from build123d import *

# Parameters (mm, degrees)
SKETCH1_W           = 230
SKETCH1_H           = 102
BOSS_EXTRUDE1_DEPTH = 2
SKETCH2_W           = 37
SKETCH2_H           = 22
SKETCH2_W_2         = 35
SKETCH2_H_2         = 9
SKETCH2_W_3         = 50
SKETCH2_H_3         = 56
CUT_EXTRUDE1_DEPTH  = 252.610810579
SKETCH3_R           = 1.65
CUT_EXTRUDE2_DEPTH  = 10
FILLET1_R           = 4
FILLET2_SIZE        = 4
FILLET2_SIZE_2      = 12
FILLET3_R           = 10
SKETCH4_R           = 1.65
CUT_EXTRUDE3_DEPTH  = 10


with BuildPart() as part:
    # Sketch1 → Boss-Extrude1 (new body)
    with BuildSketch(Plane(origin=(0, 0, 0), x_dir=(1, 0, 0), z_dir=(0, 1, 0))):
        with Locations((115, 51)):
            Rectangle(SKETCH1_W, SKETCH1_H)
    extrude(amount=BOSS_EXTRUDE1_DEPTH)

    # Sketch2 → Cut-Extrude1 (cut, through all)
    with BuildSketch(Plane(origin=(0, 2, 0), x_dir=(1, 0, 0), z_dir=(0, 1, 0))):
        with Locations((18.5, 91)):
            Rectangle(SKETCH2_W, SKETCH2_H)
        with Locations((17.5, 4.5)):
            Rectangle(SKETCH2_W_2, SKETCH2_H_2)
        with Locations((211.5, 91)):
            Rectangle(SKETCH2_W, SKETCH2_H)
        with Locations((212.5, 4.5)):
            Rectangle(SKETCH2_W_2, SKETCH2_H_2)
        with Locations((115, 28)):
            Rectangle(SKETCH2_W_3, SKETCH2_H_3)
    extrude(amount=-CUT_EXTRUDE1_DEPTH, mode=Mode.SUBTRACT)

    # Sketch3 → Cut-Extrude2 (cut)
    with BuildSketch(Plane.XZ):
        with Locations(Location((5, -14, 0), (0, 0, 270))):
            Circle(SKETCH3_R)
        with Locations(Location((5, -75, 0), (0, 0, 270))):
            Circle(SKETCH3_R)
        with Locations(Location((95, -59.5, 0), (0, 0, 270))):
            Circle(SKETCH3_R)
        with Locations(Location((135, -59.5, 0), (0, 0, 270))):
            Circle(SKETCH3_R)
        with Locations(Location((225, -14, 0), (0, 0, 270))):
            Circle(SKETCH3_R)
        with Locations(Location((225, -75, 0), (0, 0, 270))):
            Circle(SKETCH3_R)
    extrude(amount=-CUT_EXTRUDE2_DEPTH, mode=Mode.SUBTRACT)

    # Fillet1
    fillet1_edges = [part.edges().sort_by_distance(p)[0] for p in [
        (0, 1, -9),
        (230, 1, -80),
        (230, 1, -9),
        (90, 1, 0),
        (140, 1, 0),
        (0, 1, -80),
    ]]
    fillet(fillet1_edges, radius=FILLET1_R)

    # Fillet2
    # an asymmetric fillet: 12, 4 mm, written as the material it adds along each edge
    with BuildSketch(Plane(origin=(195, 2, -9), x_dir=(0, 0, 1), z_dir=(0, -1, 0))) as fillet2_piece_1:
        with BuildLine():
            Bezier((FILLET2_SIZE, 0), (0, 0), (0, -FILLET2_SIZE_2), weights=[1, 0.707106781, 1])
            Line((0, -FILLET2_SIZE_2), (0, 0))
            Line((0, 0), (FILLET2_SIZE, 0))
        make_face()
    extrude(amount=2)
    with BuildSketch(Plane(origin=(35, 2, -9), x_dir=(0, 0, 1), z_dir=(0, -1, 0))) as fillet2_piece_2:
        with BuildLine():
            Bezier((FILLET2_SIZE, 0), (0, 0), (0, FILLET2_SIZE_2), weights=[1, 0.707106781, 1])
            Line((0, FILLET2_SIZE_2), (0, 0))
            Line((0, 0), (FILLET2_SIZE, 0))
        make_face()
    extrude(amount=2)

    # Fillet3
    fillet3_edges = [part.edges().sort_by_distance(p)[0] for p in [
        (35, 1, 0),
        (195, 1, 0),
    ]]
    fillet(fillet3_edges, radius=FILLET3_R)

    # Sketch4 → Cut-Extrude3 (cut)
    with BuildSketch(Plane.XZ):
        with Locations(Location((61, -7, 0), (0, 0, 270))):
            Circle(SKETCH4_R)
        with Locations(Location((169, -7, 0), (0, 0, 270))):
            Circle(SKETCH4_R)
    extrude(amount=-CUT_EXTRUDE3_DEPTH, mode=Mode.SUBTRACT)


solid = part.part
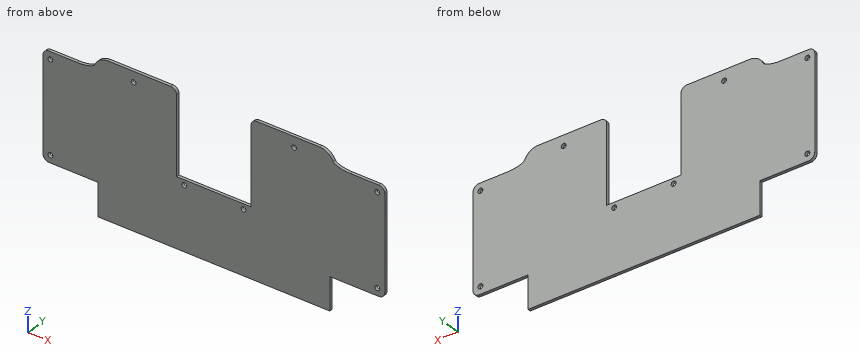
Read the model definition and answer for the solid it produces. Units are mm, in the model's axes. Round coordinates to 2 decimals unless told otherwise and drop trailing zeros. Write each loop counter-clockwise with the first axis right and the second up, starting at its lowest first coordinate (ties: lowest second). Pieces come first, ordered by that corner, then holes.
1. The part is cut by section B-B, the plane y = 1. State how many separate pieces and enclosed holes the cut face has, then the cut area to 3 significant figures.
2. The part is cut by section A-A, the plane z = -19.5. Determine the outline of the cut face in (x, y).
3. The part is cut by section C-C, the plane x = 114. Determine the outline of the cut face in (y, z), then the cut area to 3 significant figures.
4. Given pin 1 Ø0.6 at (x, y) = (219.5, 1.5) entering from +Z; pin 2 Ø1 at (x, y) = (27.5, 0.5) entering from -Z; pin 3 Ø0.6 at (y, z) = (0.5, -88) entering from -X, each flat-ended and moving along its own axis, determine where each tip first touches the part or whether it passes through.
5. Straight lines are drawn through the part: L1, parallel to X at y = 1.5, z = -75; L2, parallel to X at y = 1, z = -14; L3, parallel to Z at x = 225, y = 1.05. For each, find the intervals that lie inside material, in ascending order.
6. The part is cut by section D-D, the plane z = -88. Determine the outline of the cut face in (x, y), then the cut area to 3 significant figures.
Values:
1. separate pieces: 1
1. enclosed holes: 8
1. area: 18,300 mm2
2. outline: (0, 0) - (90, 0) - (90, 2) - (0, 2) - close; (140, 0) - (230, 0) - (230, 2) - (140, 2) - close
3. outline: (0, -102) - (2, -102) - (2, -56) - (0, -56) - close
3. area: 92.0 mm2
4. pin 1: stops at z = -9
4. pin 2: stops at z = -80
4. pin 3: stops at x = 37
5. L1: x = 0 to 3.35, 6.65 to 223.35, 226.65 to 230
5. L2: x = 0 to 3.35, 6.65 to 90, 140 to 223.35, 226.65 to 230
5. L3: z = -80 to -76.65, -73.35 to -15.65, -12.35 to -9
6. outline: (37, 0) - (193, 0) - (193, 2) - (37, 2) - close
6. area: 312 mm2
